Verification items for the finished model (mm, model axes). A direction names the side the tool comes from. Give positions to 0.01 mm unless a question says otherwise; leave off trailing zeros. Write each loop counter-clockwise with the first axis right and the second up, starting at its lowest first coordinate (ties: lowest second). Pieces come first, ordered by that corner, then holes. Notation, with made-up numbers: (86, -37) -> (137, -37) arc R24 cw to (137, -12) -> close; hole circle Ø10 at (-22.75, -28). An arc over 180 degrees is marked (long way). Answer as CSV lines item,"result". Start each with the question number.
1) Mould release check, pull along Z, two halves, no side actions. Record for faces 4 (the flat face through (7, 54, -21.844)), 5 (the cylindrical face through (27.307, -4.829, 1.294)), 6 (the flat face through (7, 35, -7.747)): released by +Z, released by -Z, zero draft, split by the parting line, or undercut.
2) Material ranges on L1, parallel to Y at x = 0, z = -14 (3 decimals); L2, parallel to Y at x = -1, z = -18.5 (3 decimals); L3, parallel to Z at x = -25, y = -5, recorded low to high.
3) Tool access check on faces 1 (the flat face through (-4.826, 12, 0)), 2 (the flat face through (21, 0, 1)), 3 (the cylindrical face through (0.53, -1.82, -18.04)). Record the directions out of +Z, -Z, +X, -X, +Y, -Y that give a thin tool (end or side, any length) a straight path to the whole face; none if there is none.
4) Gauge pin test, flat ends, axial feed: pin 1 Ø5 at (y, z) = (43, -12) entering from -X; pin 2 Ø4 at (x, y) = (-20, 40.5) entering from +Z; pin 3 Ø3 at (y, z) = (42, -11.5) entering from +X; pin 4 Ø8.5 at (y, z) = (13, 2.5) entering from +X. Record the tip position at first contact, or that the pin passes through.
5) Sectioned sample at D-D on y = 56.5. Record the cut outline in (x, z), and give its area (3 significant figures).
6) Sectioned sample at C-C on y = 1. Record the cut outline in (x, z), and give its area (3 significant figures).
7) Sectioned sample at A-A on x = 0. Record the cut outline in (y, z) (3 decimals).
8) Sectioned sample at B-B on z = 6. Record the cut outline in (x, y) (3 decimals), and give its area (3 significant figures).
```python
from build123d import *

# Parameters (mm, degrees)
SKETCH1_W                  = 76.2
SKETCH1_H                  = 39.624
BOSS_EXTRUDE1_DEPTH        = 9.525
CUT_EXTRUDE1_DEPTH         = 80.307508907
FILLET1_SIZE               = 12.7
SKETCH12_R                 = 6.35
BOSS_EXTRUDE4_DEPTH        = 9.525
BOSS_EXTRUDE5_START        = -14.097
SKETCH13_R                 = 16.002
BOSS_EXTRUDE5_DEPTH        = 14.097
SKETCH14_R                 = 6.35
CUT_EXTRUDE4_DEPTH         = 85.308297475
BOSS_EXTRUDE6_DEPTH        = 4.826
F_3_8_0_5_DIAMETER_HOLE1_D = 12.7


with BuildPart() as part:
    # Sketch1 → Boss-Extrude1 (new body)
    with BuildSketch(Plane(origin=(0, 0, 0), x_dir=(1, 0, 0), z_dir=(0, 1, 0))):
        Rectangle(SKETCH1_W, SKETCH1_H)
    extrude(amount=-BOSS_EXTRUDE1_DEPTH)

    # Sketch2 → Cut-Extrude1 (cut, through all)
    with BuildSketch(Plane(origin=(38.1, 0, 0), x_dir=(0, 0, -1), z_dir=(1, 0, 0))):
        with BuildLine():
            Line((17.272, 0), (19.812, 0))
            Line((19.812, 0), (19.812, -2.54))
            ThreePointArc((19.812, -2.54), (18.015948776, -1.796051224), (17.272, 0))
        make_face()
    extrude(amount=-CUT_EXTRUDE1_DEPTH, mode=Mode.SUBTRACT)

    # Fillet1
    # a fillet whose section is not a circle: 12.7 mm, written as the material it takes off along each edge
    with BuildSketch(Plane(origin=(-38.1, 31.75, 19.812), x_dir=(1, 0, 0), z_dir=(0, -1, 0))) as fillet1_piece_1:
        with BuildLine():
            Bezier((FILLET1_SIZE, 0), (0, 0), (0, -FILLET1_SIZE), weights=[1, 1, 1])
            Line((0, -FILLET1_SIZE), (0, 0))
            Line((0, 0), (FILLET1_SIZE, 0))
        make_face()
    extrude(amount=73.025, mode=Mode.SUBTRACT)
    with BuildSketch(Plane(origin=(38.1, 31.75, 19.812), x_dir=(-1, 0, 0), z_dir=(0, -1, 0))) as fillet1_piece_2:
        with BuildLine():
            Bezier((FILLET1_SIZE, 0), (0, 0), (0, FILLET1_SIZE), weights=[1, 1, 1])
            Line((0, FILLET1_SIZE), (0, 0))
            Line((0, 0), (FILLET1_SIZE, 0))
        make_face()
    extrude(amount=73.025, mode=Mode.SUBTRACT)

    # Sketch12 → Boss-Extrude4 (add)
    with BuildSketch(Plane.XY.offset(-17.272)):
        with BuildLine():
            Line((-16.002, 53.975), (-16.002, 16.002))
            ThreePointArc((-16.002, 16.002), (-20.688877287, 4.686877287), (-32.004, 0))
            Line((-32.004, 0), (32.004, 0))
            ThreePointArc((32.004, 0), (20.688877287, 4.686877287), (16.002, 16.002))
            Line((16.002, 16.002), (16.002, 53.975))
            ThreePointArc((16.002, 53.975), (0, 69.977), (-16.002, 53.975))
        make_face()
        with Locations(Location((0, 53.975, 0), (0, 0, 180))):
            Circle(SKETCH12_R, mode=Mode.SUBTRACT)
    extrude(amount=BOSS_EXTRUDE4_DEPTH)

    # Sketch13 → Boss-Extrude5 (add)
    with BuildSketch(Plane.XY.offset(-7.747).offset(BOSS_EXTRUDE5_START)):
        with Locations((0, 53.975)):
            Circle(SKETCH13_R)
    extrude(amount=BOSS_EXTRUDE5_DEPTH)

    # Sketch14 → Cut-Extrude4 (cut, through all)
    with BuildSketch(Plane.XY.offset(-7.747)):
        with Locations((0, 53.975)):
            Circle(SKETCH14_R)
    extrude(amount=-CUT_EXTRUDE4_DEPTH, mode=Mode.SUBTRACT)

    # Sketch15 → Boss-Extrude6 (add, symmetric)
    with BuildSketch(Plane(origin=(0, 0, 0), x_dir=(0, 0, -1), z_dir=(1, 0, 0))):
        Polygon((7.747, 0), (7.747, 41.275), (-19.812, 0), align=None)
    extrude(amount=BOSS_EXTRUDE6_DEPTH, both=True)

    # 3/8 (0.5) Diameter Hole1 (through all)
    with Locations(Plane(origin=(-25.4, 0, 7.112), x_dir=(0, 0, 1), z_dir=(0, 1, 0))):
        with Locations((0, 0), (0.238495024, 50.799440156)):
            Hole(F_3_8_0_5_DIAMETER_HOLE1_D / 2)


solid = part.part
```
Ans:
1,face 4,"released by -Z"
1,face 5,"undercut"
1,face 6,"released by +Z"
2,L1,"y = -9.525 to 47.625, 60.325 to 69.977"
2,L2,"y = -9.525 to -2.175, 38.004 to 47.704, 60.246 to 69.946"
2,L3,"z = -19.81 to 0.77, 13.45 to 19.81"
3,face 1,"+Z, -X, +Y"
3,face 2,"+Z, +X, +Y"
3,face 3,"-Z, +X, -X"
4,pin 1,"stops at x = -16"
4,pin 2,"passes through"
4,pin 3,"stops at x = 16"
4,pin 4,"stops at x = 4.83"
5,outline,"(-15.8, -21.84) -> (-5.83, -21.84) -> (-5.83, -7.75) -> (-15.8, -7.75) -> close; (5.83, -21.84) -> (15.8, -21.84) -> (15.8, -7.75) -> (5.83, -7.75) -> close"
5,area,"281 mm²"
6,outline,"(-26.44, -17.27) -> (26.44, -17.27) -> (26.44, -7.75) -> (4.83, -7.75) -> (4.83, 19.14) -> (-4.83, 19.14) -> (-4.83, -7.75) -> (-26.44, -7.75) -> close"
6,area,"763 mm²"
7,outline,"(-9.525, -19.812) -> (-2.54, -19.812) arc R2.54 cw to (0, -17.272) -> (37.973, -17.272) -> (37.973, -21.844) -> (47.625, -21.844) -> (47.625, -7.747) -> (41.275, -7.747) -> (0, 19.812) -> (-9.525, 19.812) -> close; (60.325, -21.844) -> (69.977, -21.844) -> (69.977, -7.747) -> (60.325, -7.747) -> close"
8,outline,"(-38.1, -9.525) -> (-31.652, -9.525) -> (-31.652, 0) -> (-38.1, 0) -> close; (-19.148, -9.525) -> (19.195, -9.525) -> (19.195, 0) -> (4.826, 0) -> (4.826, 20.686) -> (-4.826, 20.686) -> (-4.826, 0) -> (-19.148, 0) -> close; (31.604, -9.525) -> (38.1, -9.525) -> (38.1, 0) -> (31.604, 0) -> close"
8,area,"688 mm²"
